Verification items for this drawing (mm, ordinates from the low corner). Coordinates: 2 decimals unless noted, no trailing zeros. Loops run counter-clockwise (first coordinate to the right, second up) from the corner with the lowest first, then second, coordinate; pieces in that order, holes last. Notation, with made-up numbers: M -18,67 L 12,67 A33 cw 12,95 Z; hole C 13.5,28.5 d3. An arc over 180 degrees is marked long. One line per question, with ' | ' between items. Start each with the question number.
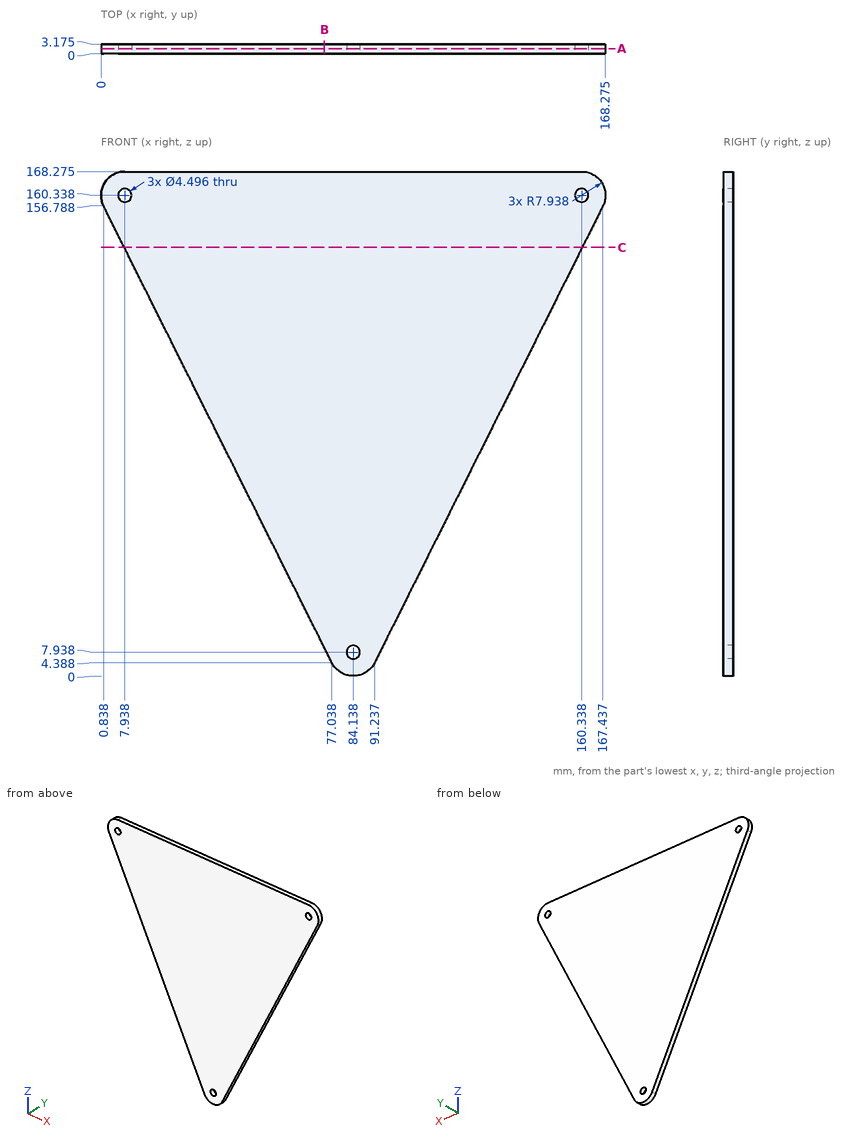
1. Sectioned sample at B-B (x = 74.5). Record the cut outline in (y, z) (1 decimal).
2. Sectioned sample at A-A (y = 1.6). Record the cut outline in (x, z) (1 decimal).
3. Thickness scan on line 1 (Z direction, x = 7.5, y = 0.75) (1 decimal); line 2 (X direction, y = 1.8, z = 142.5) (1 decimal); line 3 (Z direction, x = 25, y = 2.2) (1 decimal). Record the ranges inside material, lowest first.
4. Depth check by flat-ended pin: pin 1 Ø2.5 at (x, z) = (84.14, 7.94) entering from -Y. Enter the tip coordinate at first touch or a pass-through.
5. Sectioned sample at C-C (z = 143). Record the cut outline in (x, y) (1 decimal), and give its area (3 significant figures).
Result:
1) outline: M 0,9.5 L 3.2,9.5 L 3.2,168.3 L 0,168.3 Z
2) outline: M 0.8,156.8 L 77,4.4 A7.9 ccw 91.2,4.4 L 167.4,156.8 A7.9 ccw 160.3,168.3 L 7.9,168.3 A7.9 ccw Z; hole C 7.9,160.3 d4.5; hole C 84.1,7.9 d4.5; hole C 160.3,160.3 d4.5
3) line 1: z = 143.5 to 158.1, 162.5 to 168.3 | line 2: x = 8 to 160.3 | line 3: z = 108.5 to 168.3
4) pin 1: passes through
5) outline: M 7.7,0 L 160.5,0 L 160.5,3.2 L 7.7,3.2 Z | area: 485 mm2
